from build123d import *

# Parameters (mm, degrees)
F0_R      = 59.253304
F1_DEPTH  = 25.4
F2_R      = 54.171653
F3_DEPTH  = 25.4
F4_R      = 46.400893
F5_DEPTH  = 25.4
F6_R      = 38.807886
F7_DEPTH  = 25.4
F8_R      = 30.841297
F9_DEPTH  = 25.4
F10_R     = 22.983949
F11_DEPTH = 25.4
F12_R     = 16.943249
F13_DEPTH = 25.4


with BuildPart() as f1:
    # F0 (on Front) → F1 (new body)
    with BuildSketch(Plane.XZ):
        Circle(F0_R)
    extrude(amount=F1_DEPTH)

    # F2 (on face) → F3 (join)
    with BuildSketch(Plane.XZ.offset(25.4)):
        Circle(F2_R)
    extrude(amount=F3_DEPTH)

    # F4 (on face) → F5 (join)
    with BuildSketch(Plane.XZ.offset(50.8)):
        Circle(F4_R)
    extrude(amount=F5_DEPTH)

    # F6 (on face) → F7 (join)
    with BuildSketch(Plane.XZ.offset(76.2)):
        Circle(F6_R)
    extrude(amount=F7_DEPTH)

    # F8 (on face) → F9 (join)
    with BuildSketch(Plane.XZ.offset(101.6)):
        Circle(F8_R)
    extrude(amount=F9_DEPTH)

    # F10 (on face) → F11 (join)
    with BuildSketch(Plane.XZ.offset(127)):
        Circle(F10_R)
    extrude(amount=F11_DEPTH)

    # F12 (on face) → F13 (join)
    with BuildSketch(Plane.XZ.offset(152.4)):
        Circle(F12_R)
    extrude(amount=F13_DEPTH)


solid = f1.part
Verification items for the finished model (mm, model axes). A direction names the side the tool comes from. Round coordinates to 2 decimals unless told otherwise and drop trailing zeros. Order: outer loops, then holes, each group sorted by start corner. A loop starts at its lowest first (then second) coordinate and runs counter-clockwise, first axis right, second up.
1. Section check D-D on x = 51. Record the cut outline in (y, z), then the cut area to 3 significant figures.
Final values:
outline: (-50.8, -18.26) - (-25.4, -18.26) - (-25.4, -30.17) - (0, -30.17) - (0, 30.17) - (-25.4, 30.17) - (-25.4, 18.26) - (-50.8, 18.26) - close
area: 2,460 mm2
2. Section check A-A on z = 0. Record the cut outline in (x, y).
Final values:
outline: (-59.25, -25.4) - (-54.17, -25.4) - (-54.17, -50.8) - (-46.4, -50.8) - (-46.4, -76.2) - (-38.81, -76.2) - (-38.81, -101.6) - (-30.84, -101.6) - (-30.84, -127) - (-22.98, -127) - (-22.98, -152.4) - (-16.94, -152.4) - (-16.94, -177.8) - (16.94, -177.8) - (16.94, -152.4) - (22.98, -152.4) - (22.98, -127) - (30.84, -127) - (30.84, -101.6) - (38.81, -101.6) - (38.81, -76.2) - (46.4, -76.2) - (46.4, -50.8) - (54.17, -50.8) - (54.17, -25.4) - (59.25, -25.4) - (59.25, 0) - (-59.25, 0) - close
3. Go/stop test with flat-tipped pins: P1, Ø2, axis at x = -14.5, y = -76.5, coming from the -Z side; P2, Ø10, axis at x = -13.5, z = 46, coming from the -Y side; P3, Ø10, axis at x = 26, y = -100, coming from the +Z side. Record where each tip stops, or that it passes through.
Final values:
P1: stops at z = -44.38
P2: stops at y = -76.2
P3: stops at z = 32.64
4. Access from +Z, -Z, +X, -X, +Y, -Y to the whole of each face (thin tool, end or side, straight path). Record for faces 1 (the flat face through (-11, -76.2, -38)), 2 (the flat face through (0, -177.8, 0)).
Final values:
face 1: -Y
face 2: +Z, -Z, +X, -X, -Y
5. Section check C-C on y = -39. Record the cut outline in (x, z), then the cut area to 3 significant figures.
Final values:
outline: circle Ø108.34 at (0, 0)
area: 9,220 mm2
6. Thickness scan on L1, parallel to Z at x = -24, y = -16; L2, parallel to Y at x = 18, z = -42.5; L3, parallel to Y at x = 3.5, z = -51. Record the ranges inside material, lowest first.
Final values:
L1: z = -54.18 to 54.18
L2: y = -76.2 to 0
L3: y = -50.8 to 0
7. Section check B-B on x = 0. Record the cut outline in (y, z).
Final values:
outline: (-177.8, -16.94) - (-152.4, -16.94) - (-152.4, -22.98) - (-127, -22.98) - (-127, -30.84) - (-101.6, -30.84) - (-101.6, -38.81) - (-76.2, -38.81) - (-76.2, -46.4) - (-50.8, -46.4) - (-50.8, -54.17) - (-25.4, -54.17) - (-25.4, -59.25) - (0, -59.25) - (0, 59.25) - (-25.4, 59.25) - (-25.4, 54.17) - (-50.8, 54.17) - (-50.8, 46.4) - (-76.2, 46.4) - (-76.2, 38.81) - (-101.6, 38.81) - (-101.6, 30.84) - (-127, 30.84) - (-127, 22.98) - (-152.4, 22.98) - (-152.4, 16.94) - (-177.8, 16.94) - close
